The model under review builds one solid part; all positions refer to its coordinate system, in mm. Coordinates: 2 decimals unless noted, no trailing zeros. Order: outer loops, then holes, each group sorted by start corner. A loop starts at its lowest first (then second) coordinate and runs counter-clockwise, first axis right, second up.
Autodesk Inventor part; units mm, degrees
ref_plane "YZ Plane" through (0, 0, 0) normal (1, 0, 0) x (0, 1, 0)
ref_plane "XZ Plane" through (0, 0, 0) normal (0, 1, 0) x (-1, 0, 0)
ref_plane "XY Plane" through (0, 0, 0) normal (0, 0, 1) x (1, 0, 0)
sketch "Sketch1" plane through (0, 0, 0) normal (0, 0, 1) x (1, 0, 0)
  circle A0 centre (0, 0) radius 10
  circle A1 centre (0, 0) radius 8
  dimension "d0" = 16
  dimension "d1" = 20
extrude "Extrusion1" add sketch "Sketch1" along normal blind 300
sketch "Sketch2" plane through (0, 0, 0) normal (0, 1, 0) x (-1, 0, 0)
  line L0 (1.5, 8) -> (-1.5, 8)
  line L1 (-1.5, 8) -> (-1.5, 24)
  line L2 (-1.5, 24) -> (1.5, 24)
  line L3 (1.5, 24) -> (1.5, 8)
  line L4 (-1.5, 46.9938) -> (-10, 46.9938)
  line L5 (-10, 0) -> (-10, 300)
  line L6 (1.5, 47.6647) -> (10, 47.6647)
  line L7 (10, 0) -> (10, 300)
  line L8 (10, 0) -> (-10, 0)
  line L9 (1.5, 40) -> (-1.5, 40)
  line L10 (-1.5, 40) -> (-1.5, 56)
  line L11 (-1.5, 56) -> (1.5, 56)
  line L12 (1.5, 56) -> (1.5, 40)
  point P0 (0, 0)
  dimension "d4" = 3
  dimension "d5" = 16
  dimension "d6" = 8
  dimension "d7" = 16
  dimension "d8" = 3
  dimension "d9" = 16
extrude "Extrusion2" cut sketch "Sketch2" along normal through all both and the other way through all contours L0 L1 L2 L3 | L10 L11 L12 L9
sketch "Sketch3" plane through (0, 0, 0) normal (1, 0, 0) x (0, 1, 0)
  line L0 (1.5, 8) -> (-1.5, 8)
  line L1 (-1.5, 8) -> (-1.5, 24)
  line L2 (-1.5, 24) -> (1.5, 24)
  line L3 (1.5, 24) -> (1.5, 8)
  line L4 (-1.5, 46.9938) -> (-10, 46.9938)
  line L5 (1.5, 47.6647) -> (10, 47.6647)
  line L6 (10, 0) -> (-10, 0)
  line L7 (1.5, 40) -> (-1.5, 40)
  line L8 (-1.5, 40) -> (-1.5, 56)
  line L9 (-1.5, 56) -> (1.5, 56)
  line L10 (1.5, 56) -> (1.5, 40)
  line L11 (1.5, 18.1726) -> (10, 18.1726)
  line L12 (10, 0) -> (10, 300)
  line L13 (-1.5, 20.0085) -> (-10, 20.0085)
  line L14 (-10, 0) -> (-10, 300)
  point P0 (0, 0)
  point P1 (0, 0)
  dimension "d12" = 3
  dimension "d13" = 16
  dimension "d15" = 16
  dimension "d16" = 3
  dimension "d17" = 16
  dimension "d18" = 8
extrude "Extrusion3" cut sketch "Sketch3" along normal through all both and the other way through all contours L0 L1 L2 L3 | L10 L7 L8 L9
equation "\"BendRadius\" = Thickness"
equation "\"BendReliefWidth\" = Thickness"
equation "\"BendReliefDepth\" = 0.5 * Thickness"
equation "\"CornerReliefSize\" = 4 * Thickness"
equation "\"MinimumRemnant\" = 2 * Thickness"
equation "\"TransitionRadius\" = BendRadius"
equation "\"JacobiRadiusSize\" = BendRadius"
equation "\"GapSize\" = Thickness"
properties part number "tail" material "PVC-Piping"
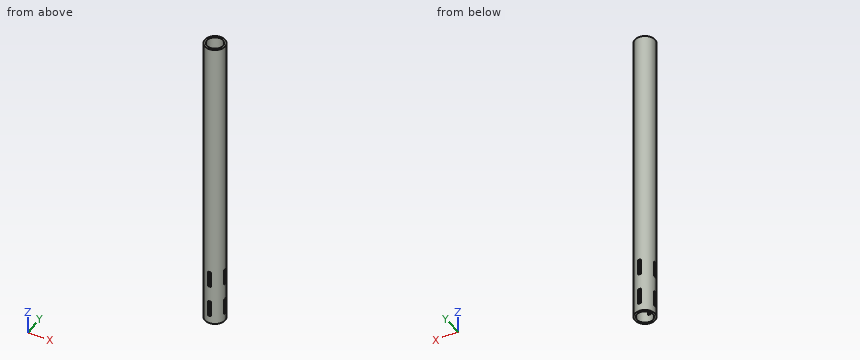
(1) Consider section B-B (z = 161). Give the boundary of the cut face in (x, y), then the cut area to 3 significant figures.
(2) Consider section A-A (y = 4.75). Give the boundary of the cut face in (x, z).
(3) Insertion check: pin 1 Ø5 at (y, z) = (6, 153) entering from +X; pin 2 Ø3 at (x, y) = (0, -5) entering from +Z; pin 3 Ø6 at (x, z) = (0.5, 52.5) entering from -Y; pin 4 Ø1.6 at (y, z) = (-9, 12.5) entering from -X. Each pin has a flat end and moves straight along its axis. Give the tip position at first contact, or say it passes through.
(4) Wall thickness on line 1 (Z direction, x = 8.75, y = -1); line 2 (Y direction, x = 0, z = 124.5); line 3 (X direction, y = -0.75, z = 84): over which ranges is each line inside the solid? List them lowest first.
Findings:
1. outline: circle Ø20 at (0, 0); hole circle Ø16 at (0, 0)
1. area: 113 mm2
2. outline: (-8.8, 0) - (-6.44, 0) - (-6.44, 300) - (-8.8, 300) - close; (6.44, 0) - (8.8, 0) - (8.8, 300) - (6.44, 300) - close
3. pin 1: stops at x = 9.37
3. pin 2: passes through
3. pin 3: stops at y = -9.89
3. pin 4: stops at x = -5.72
4. line 1: z = 0 to 8, 24 to 40, 56 to 300
4. line 2: y = -10 to -8, 8 to 10
4. line 3: x = -9.97 to -7.96, 7.96 to 9.97
